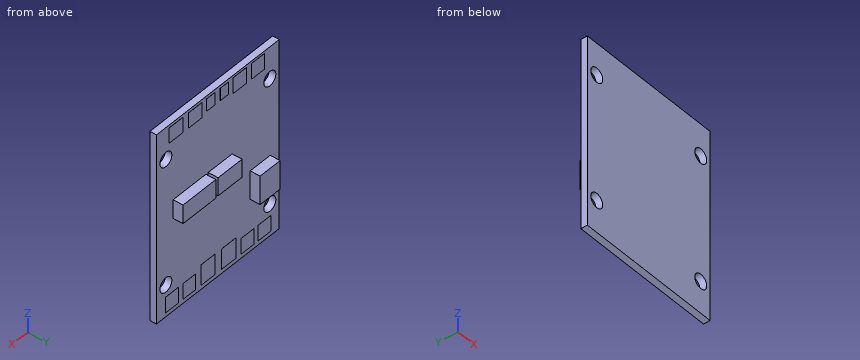
```python
from build123d import *

# Parameters (mm, degrees)
SKETCH1_W        = 36
SKETCH1_H        = 5
SKETCH1_H_2      = 36
SKETCH1_R        = 1.75
PCB_DEPTH        = 1.6
SKETCH4_W        = 3.740798036
SKETCH4_H        = 3.820815106
SKETCH4_W_2      = 3.820815106
SKETCH4_W_3      = 4.160887655
SKETCH4_H_2      = 4.981062625
SKETCH4_W_4      = 4.100874852
SKETCH4_W_5      = 3.695656728
SKETCH4_W_6      = 3.812361676
SKETCH4_W_7      = 3.787546171
SKETCH4_H_3      = 3.830762868
SKETCH4_W_8      = 4.01762935
SKETCH4_W_9      = 2.467816827
SKETCH4_H_4      = 3.027236998
SKETCH4_W_10     = 2.483275044
SKETCH4_W_11     = 3.953731944
SKETCH4_H_5      = 3.718642979
SKETCH4_W_12     = 4.022264052
PADS_DEPTH       = 0.01
SKETCH2_W        = 5.863870515
SKETCH2_H        = 6.933382723
SKETCH2_W_2      = 7.016073618
SKETCH2_H_2      = 4.389541424
SKETCH2_W_3      = 9.613875512
SKETCH2_H_3      = 4.530712508
COMPONENTS_DEPTH = 2.4


with BuildPart() as part:
    # Sketch1 → PCB (new body)
    # profile 1 of 3: a face of its own
    with BuildSketch(Plane(origin=(0, 0, 0), x_dir=(1, 0, 0), z_dir=(0, 1, 0))):
        with Locations((0, 20.5)):
            Rectangle(SKETCH1_W, SKETCH1_H)
    # profile 2 of 3: a face of its own
    with BuildSketch(Plane(origin=(0, 0, 0), x_dir=(1, 0, 0), z_dir=(0, 1, 0))):
        Rectangle(SKETCH1_W, SKETCH1_H_2)
        with Locations(Location((-15.25, -15.25, 0), (0, 0, 270))):
            Circle(SKETCH1_R, mode=Mode.SUBTRACT)
        with Locations(Location((15.25, -15.25, 0), (0, 0, 270))):
            Circle(SKETCH1_R, mode=Mode.SUBTRACT)
        with Locations(Location((-15.25, 15.25, 0), (0, 0, 270))):
            Circle(SKETCH1_R, mode=Mode.SUBTRACT)
        with Locations(Location((15.25, 15.25, 0), (0, 0, 270))):
            Circle(SKETCH1_R, mode=Mode.SUBTRACT)
    # profile 3 of 3: a face of its own
    with BuildSketch(Plane(origin=(0, 0, 0), x_dir=(1, 0, 0), z_dir=(0, 1, 0))):
        with Locations((0, -20.5)):
            Rectangle(SKETCH1_W, SKETCH1_H)
    extrude(amount=PCB_DEPTH)

    # Sketch4 → Pads (add)
    with BuildSketch(Plane(origin=(0, 1.6, 0), x_dir=(1, 0, 0), z_dir=(0, 1, 0))):
        with Locations((-13.696501098, 20.107722338)):
            Rectangle(SKETCH4_W, SKETCH4_H)
        with Locations((-8.65542567, 20.107722338)):
            Rectangle(SKETCH4_W_2, SKETCH4_H)
        with Locations((-3.164254223, 19.527598579)):
            Rectangle(SKETCH4_W_3, SKETCH4_H_2)
        with Locations((2.907040985, 19.527598579)):
            Rectangle(SKETCH4_W_4, SKETCH4_H_2)
        with Locations((8.437153549, 20.107722338)):
            Rectangle(SKETCH4_W_5, SKETCH4_H)
        with Locations((13.494368018, 20.107722338)):
            Rectangle(SKETCH4_W_6, SKETCH4_H)
        with Locations((-11.802728013, -20.491019937)):
            Rectangle(SKETCH4_W_7, SKETCH4_H_3)
        with Locations((-6.386521753, -20.491019937)):
            Rectangle(SKETCH4_W_8, SKETCH4_H_3)
        with Locations((-1.930345809, -20.780662983)):
            Rectangle(SKETCH4_W_9, SKETCH4_H_4)
        with Locations((2.098241081, -20.780662983)):
            Rectangle(SKETCH4_W_10, SKETCH4_H_4)
        with Locations((6.660299296, -20.434959993)):
            Rectangle(SKETCH4_W_11, SKETCH4_H_5)
        with Locations((12.296113939, -20.434959993)):
            Rectangle(SKETCH4_W_12, SKETCH4_H_5)
    extrude(amount=PADS_DEPTH)

    # Sketch2 → Components (add)
    with BuildSketch(Plane(origin=(0, 1.6, 0), x_dir=(1, 0, 0), z_dir=(0, 1, 0))):
        with Locations((-12.422852881, 6.938659117)):
            Rectangle(SKETCH2_W, SKETCH2_H)
        with Locations((-0.676707896, -1.879325534)):
            Rectangle(SKETCH2_W_2, SKETCH2_H_2)
        with Locations((8.311019041, -1.808739992)):
            Rectangle(SKETCH2_W_3, SKETCH2_H_3)
    extrude(amount=COMPONENTS_DEPTH)


solid = part.part
```
Here's how the part is built. I have some questions about the finished solid (model axes, mm). Give positions to 0.01 mm unless a question says otherwise; leave off trailing zeros. Write each loop counter-clockwise with the first axis right and the second up, starting at its lowest first coordinate (ties: lowest second). Pieces come first, ordered by that corner, then holes. Notation, with made-up numbers: M 12.5,21.5 L 40.5,21.5 A20 cw 40.5,34.5 Z; hole C -24,6 d6. An arc over 180 degrees is marked long. Put each result on its own line as item: value. Start each with the question number.
Item 1: If we section it at D-D, the plane z = -8: Write out the boundary of the cut face in (x, y), then the cut area to 3 significant figures.
Item 2: If we section it at A-A, the plane z = 15.25: Write out the boundary of the cut face in (x, y).
Item 3: I need wall thicknesses on L1, parallel to X at y = 0.65, z = -15.25; L2, parallel to X at y = 2.8, z = 2.5; L3, parallel to Y at x = 15.5, z = 18.5. Which ranges of each line are inside material? Lowest first, please. Write a range as from..to.
Item 4: Will these pins go through, and if not, where does the flat tip stop? pin 1 (3 mm diameter, centred on x = 15.25, z = 15.25, fed in from -Y); pin 2 (1.2 mm diameter, centred on y = 2.5, z = 0.5, fed in from +X); pin 3 (4 mm diameter, centred on x = 8, z = -21, fed in from +Y).
Item 5: If we section it at B-B, the plane y = 2.4: Write out the boundary of the cut face in (x, z), then the cut area to 3 significant figures.
Values:
1. outline: M -18,0 L 18,0 L 18,1.6 L -9.49,1.6 L -9.49,4 L -15.35,4 L -15.35,1.6 L -18,1.6 Z
1. area: 71.7 mm²
2. outline: M -18,0 L -17,0 L -17,1.6 L -18,1.6 Z; M -13.5,0 L 13.5,0 L 13.5,1.6 L -13.5,1.6 Z; M 17,0 L 18,0 L 18,1.6 L 17,1.6 Z
3. L1: -18..-17, -13.5..13.5, 17..18
3. L2: -4.18..2.83, 3.5..13.12
3. L3: 0..1.6
4. pin 1: through
4. pin 2: x = 13.12
4. pin 3: y = 1.61
5. outline: M -15.35,-10.41 L -9.49,-10.41 L -9.49,-3.47 L -15.35,-3.47 Z; M -4.18,-0.32 L 2.83,-0.32 L 2.83,4.07 L -4.18,4.07 Z; M 3.5,-0.46 L 13.12,-0.46 L 13.12,4.07 L 3.5,4.07 Z
5. area: 115 mm²
